```python
from build123d import *

# Parameters (mm, degrees)
BOSS_EXTRUDE1_DEPTH   = 115
RIB3_REACH            = 65.028
SKETCH4_WALL_W        = 145.325459352
SKETCH4_WALL_H        = 3
RIB4_START            = -3
RIB4_DEPTH            = 3
F_6_CLEARANCE_HOLE1_D = 3.7973
SKETCH6_R             = 2.3495
CUT_EXTRUDE1_DEPTH    = 7
SKETCH12_R            = 2.6162
CUT_EXTRUDE2_DEPTH    = 6.35


# Read off the part's stored shape, not the designer's step: Rib4
with BuildPart() as part:
    # Sketch1 → Boss-Extrude1 (new body)
    with BuildSketch(Plane.XY):
        with BuildLine():
            Line((0, 0), (0, 9.5))
            Line((0, 9.5), (-8, 9.5))
            Line((-8, 9.5), (-8, 6))
            ThreePointArc((-8, 6), (-8.878679656, 3.878679656), (-11, 3))
            Line((-11, 3), (-24, 3))
            Line((-24, 3), (-24, 0))
            Line((-24, 0), (0, 0))
        make_face()
    extrude(amount=BOSS_EXTRUDE1_DEPTH)

    # Sketch4 wall → Rib3 (add, up to next)
    with BuildSketch(Plane(origin=(-16, 6.25, 57.5), x_dir=(-0.926466577122, -0.376377046956, 0), z_dir=(-0.376377046956, 0.926466577122, 0)), mode=Mode.PRIVATE) as rib3_sk1:
        Rectangle(SKETCH4_WALL_W, SKETCH4_WALL_H)
    rib3_tool1 = extrude(rib3_sk1.sketch, amount=-RIB3_REACH, mode=Mode.PRIVATE) - part.part
    add(rib3_tool1.solids().sort_by_distance((-16, 6.25, 57.5))[0])

    # Rib4 outline → Rib4 (add)
    with BuildSketch(Plane(origin=(0, 0, 0), x_dir=(-1, 0, 0), z_dir=(0, 0, -1)).offset(RIB4_START)):
        with BuildLine():
            Line((24, 3), (8, 9.5))
            Line((8, 9.5), (8, 6))
            ThreePointArc((8, 6), (8.878679656, 3.878679656), (11, 3))
            Line((11, 3), (24, 3))
        make_face()
    rib4 = extrude(amount=RIB4_DEPTH)

    # Mirror1: Rib4 across plane
    add(rib4.mirror(Plane(origin=(0, 0, 57.5), x_dir=(1, 0, 0), z_dir=(0, 0, -1))))

    # #6 Clearance Hole1 (through all)
    with Locations(Plane(origin=(0, 0, 0), x_dir=(-1, 0, 0), z_dir=(0, -1, 0))):
        with Locations((17.5, -30), (17.5, -85)):
            Hole(F_6_CLEARANCE_HOLE1_D / 2)

    # Sketch6 → Cut-Extrude1 (cut)
    with BuildSketch(Plane(origin=(0, 0, 0), x_dir=(0, 0, -1), z_dir=(1, 0, 0))):
        with Locations((-85, 4.75)):
            Circle(SKETCH6_R)
        with Locations((-30, 4.75)):
            Circle(SKETCH6_R)
    extrude(amount=-CUT_EXTRUDE1_DEPTH, mode=Mode.SUBTRACT)

    # Sketch12 → Cut-Extrude2 (cut)
    with BuildSketch(Plane(origin=(0, 0, 0), x_dir=(0, 0, -1), z_dir=(1, 0, 0))):
        with Locations((-85, 4.75)):
            Circle(SKETCH12_R)
        with Locations((-30, 4.75)):
            Circle(SKETCH12_R)
    extrude(amount=-CUT_EXTRUDE2_DEPTH, mode=Mode.SUBTRACT)


solid = part.part
```
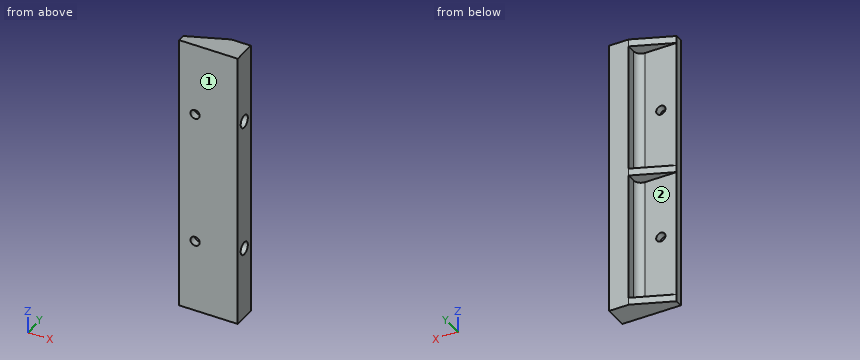
The listing builds one solid part. Answer for the finished solid, in the listing's coordinates (mm). Face numbers are marked on the shaded views. A direction names the side the tool comes from. Give positions to 0.01 mm unless a question says otherwise; leave off trailing zeros. Order: outer loops, then holes, each group sorted by start corner. A loop starts at its lowest first (then second) coordinate and runs counter-clockwise, first axis right, second up. Notation, with made-up numbers: (36, -19) -> (68, -19) arc R33 cw to (68, 13) -> close; hole circle Ø5 at (66, 30). An arc over 180 degrees is marked (long way). Answer as a JSON object with one key per item and string values. Group by question number.
Item 1: The part is cut by section D-D on x = -9. Write down the section's boundary in (y, z).
Item 2: The part is cut by section B-B on x = -17.5. Write down the section's boundary in (y, z), and give its area (3 significant figures).
Item 3: The part is cut by section C-C on z = 72. Write down the section's boundary in (x, y), and give its area (3 significant figures).
Item 4: The part is cut by section A-A on z = 85. Write down the section's boundary in (x, y).
Item 5: Flat-ended cylindrical pins translate along their axes: pin 1 (3 mm diameter, centred on y = 8.5, z = 97.5, fed in from -X); pin 2 (3 mm diameter, centred on y = 4.75, z = 85, fed in from -X); pin 3 (4 mm diameter, centred on x = -14.5, z = 25, fed in from +Y); pin 4 (3 mm diameter, centred on x = -17.5, z = 85, fed in from +Y). Find the tip coordinate at first contact, or state that the pin passes through.
Item 6: Consider L1, parallel to Z at x = -9.5, y = 6.5; L2, parallel to Z at x = -17.5, y = 0.75; L3, parallel to Y at x = -3.5, z = 85. Determine where each line is inside the solid, lowest interval first. Write a range as from..to.
Item 7: A tool of negligible diameter and unlimited length cuts with its end or side. For the marked faces 1 and 2, from which of +Z, -Z, +X, -X, +Y, -Y can it reach the whole face along a straight path? Write none if from no direction.
Result set:
{
 "1": {"outline": "(0, 0) -> (9.09, 0) -> (9.09, 3) -> (3.76, 3) -> (3.76, 56) -> (9.09, 56) -> (9.09, 59) -> (3.76, 59) -> (3.76, 112) -> (9.09, 112) -> (9.09, 115) -> (0, 115) -> close"},
 "2": {"outline": "(0, 0) -> (5.64, 0) -> (5.64, 3) -> (3, 3) -> (3, 28.1) -> (0, 28.1) -> close; (0, 31.9) -> (3, 31.9) -> (3, 56) -> (5.64, 56) -> (5.64, 59) -> (3, 59) -> (3, 83.1) -> (0, 83.1) -> close; (0, 86.9) -> (3, 86.9) -> (3, 112) -> (5.64, 112) -> (5.64, 115) -> (0, 115) -> close", "area": "346 mm²"},
 "3": {"outline": "(-24, 0) -> (0, 0) -> (0, 9.5) -> (-8, 9.5) -> (-8, 6) arc R3 cw to (-11, 3) -> (-24, 3) -> close", "area": "126 mm²"},
 "4": {"outline": "(-24, 0) -> (-19.4, 0) -> (-19.4, 3) -> (-24, 3) -> close; (-15.6, 0) -> (0, 0) -> (0, 2.13) -> (-6.35, 2.13) -> (-6.35, 2.4) -> (-7, 2.4) -> (-7, 7.1) -> (-6.35, 7.1) -> (-6.35, 7.37) -> (0, 7.37) -> (0, 9.5) -> (-8, 9.5) -> (-8, 6) arc R3 cw to (-11, 3) -> (-15.6, 3) -> close"},
 "5": {"pin 1": "x = -8", "pin 2": "x = -9.8", "pin 3": "y = 3", "pin 4": "through"},
 "6": {"L1": "0..3, 56..59, 112..115", "L2": "0..28.1, 31.9..83.1, 86.9..115", "L3": "0..2.13, 7.37..9.5"},
 "7": {"face 1": "+Z, -Z, +X, -X, -Y", "face 2": "-X, +Y"}
}
